Geometry: final body of the model. Coordinates: model frame, mm. A direction names the side the tool comes from. Give positions to 0.01 mm unless a question says otherwise; leave off trailing zeros. Loops run counter-clockwise (first coordinate to the right, second up) from the corner with the lowest first, then second, coordinate; pieces in that order, holes last. Notation, with made-up numbers: (11, 30.25) -> (70, 30.25) arc R21 ccw to (70, 39.25) -> close; hole circle Ø9 at (81.25, 61.5). An arc over 180 degrees is marked (long way). Answer in a Markdown table with one row per item. Add a question column.
from build123d import *

# Parameters (mm, degrees)
F0_W     = 609.6
F0_H     = 609.6
F0_W_2   = 406.4
F0_H_2   = 304.8
F1_DEPTH = 609.6
F2_W     = 609.6
F2_H     = 609.6
F2_W_2   = 571.5
F2_H_2   = 571.5
F3_DEPTH = 3.175
F4_W     = 412.75
F4_H     = 311.15
F4_W_2   = 406.4
F4_H_2   = 304.8
F5_DEPTH = 19.05
F6_W     = 412.75
F6_H     = 311.15
F6_W_2   = 406.4
F6_H_2   = 304.8
F7_DEPTH = 19.05


with BuildPart() as f1:
    # F0 (on Front) → F1 (new body)
    with BuildSketch(Plane.XZ):
        with Locations((-304.8, 304.8)):
            Rectangle(F0_W, F0_H)
        with Locations((-304.8, 304.8)):
            Rectangle(F0_W_2, F0_H_2, mode=Mode.SUBTRACT)
    extrude(amount=-F1_DEPTH)

    # F2 (on face) → F3 (cut)
    with BuildSketch(Plane.XY.offset(609.6)):
        with Locations((-304.8, 304.8)):
            Rectangle(F2_W, F2_H)
        with Locations((-304.8, 304.8)):
            Rectangle(F2_W_2, F2_H_2, mode=Mode.SUBTRACT)
    extrude(amount=-F3_DEPTH, mode=Mode.SUBTRACT)

    # F4 (on face) → F5 (cut)
    with BuildSketch(Plane.XZ):
        with Locations((-304.8, 304.8)):
            Rectangle(F4_W, F4_H)
        with Locations((-304.8, 304.8)):
            Rectangle(F4_W_2, F4_H_2, mode=Mode.SUBTRACT)
    extrude(amount=-F5_DEPTH, mode=Mode.SUBTRACT)

    # F6 (on face) → F7 (cut)
    with BuildSketch(Plane(origin=(0, 609.6, 0), x_dir=(-1, 0, 0), z_dir=(0, 1, 0))):
        with Locations((304.8, 304.8)):
            Rectangle(F6_W, F6_H)
        with Locations((304.8, 304.8)):
            Rectangle(F6_W_2, F6_H_2, mode=Mode.SUBTRACT)
    extrude(amount=-F7_DEPTH, mode=Mode.SUBTRACT)


solid = f1.part
(1) Cut plane B-B on z = 437.5. Return the cut outline in (x, y) (3 decimals).
(2) Reachability of faces 1 (the flat face through (-302, 600, 149.225)), 2 (the flat face through (-98.425, 9, 303)), 3 (the flat face through (-308, 301, 152.4)) from +Z, -Z, +X, -X, +Y, -Y: full face, straight path, thin tool, end or side. Return the list, or none.
(3) Material intervals for line 1 along X through (y, z) = (86.5, 202); line 2 along Z through (x, y) = (-433, 515.5), sorted ascending. Write a range as from..to.
(4) Cut plane A-A on x = -146. Return the cut outline in (y, z) (3 decimals).
(5) Pin query (flat end, axial travel): pin 1 Ø1 at (y, z) = (208.5, 607.5) entering from +X; pin 2 Ø3.5 at (x, z) = (-422, 608.5) entering from +Y; pin 3 Ø15 at (x, y) = (-305, 9.5) entering from +Z (3 decimals). Return the tip coordinate at first contact, or that it passes through.
(6) Cut plane C-C on y = 139.5. Return the cut outline in (x, z) (3 decimals), then the cut area to 3 significant figures.
(7) Draft query along Z for faces 4 (the flat face through (-309, 301, 0)), 5 (the flat face through (-302, 600, 460.375)), 6 (the flat face through (0, 301, 299)), 7 (the flat face through (-101.6, 301, 303)). Return one class per face: +Z half, -Z half, draft (parallel to the pull), parting line (faces both ways), or undercut.
Answer list:
| question | item | result |
|---|---|---|
| 1 | outline | (-609.6, 0) -> (-511.175, 0) -> (-511.175, 19.05) -> (-508, 19.05) -> (-508, 590.55) -> (-511.175, 590.55) -> (-511.175, 609.6) -> (-609.6, 609.6) -> close; (-101.6, 19.05) -> (-98.425, 19.05) -> (-98.425, 0) -> (0, 0) -> (0, 609.6) -> (-98.425, 609.6) -> (-98.425, 590.55) -> (-101.6, 590.55) -> close |
| 2 | face 1 | +Y |
| 2 | face 2 | -Y |
| 2 | face 3 | +Y, -Y |
| 3 | line 1 | x = -609.6..-508, -101.6..0 |
| 3 | line 2 | z = 0..152.4, 457.2..609.6 |
| 4 | outline | (0, 0) -> (609.6, 0) -> (609.6, 149.225) -> (590.55, 149.225) -> (590.55, 152.4) -> (19.05, 152.4) -> (19.05, 149.225) -> (0, 149.225) -> close; (0, 460.375) -> (19.05, 460.375) -> (19.05, 457.2) -> (590.55, 457.2) -> (590.55, 460.375) -> (609.6, 460.375) -> (609.6, 606.425) -> (590.55, 606.425) -> (590.55, 609.6) -> (19.05, 609.6) -> (19.05, 606.425) -> (0, 606.425) -> close |
| 5 | pin 1 | stops at x = -19.05 |
| 5 | pin 2 | stops at y = 590.55 |
| 5 | pin 3 | stops at z = 606.425 |
| 6 | outline | (-609.6, 0) -> (0, 0) -> (0, 606.425) -> (-19.05, 606.425) -> (-19.05, 609.6) -> (-590.55, 609.6) -> (-590.55, 606.425) -> (-609.6, 606.425) -> close; hole (-508, 152.4) -> (-101.6, 152.4) -> (-101.6, 457.2) -> (-508, 457.2) -> close |
| 6 | area | 248,000 mm² |
| 7 | face 4 | -Z half |
| 7 | face 5 | undercut |
| 7 | face 6 | draft |
| 7 | face 7 | undercut |
